Work out the finished part from the listing and answer in its coordinate system (mm). A direction names the side the tool comes from. Round coordinates to 2 decimals unless told otherwise and drop trailing zeros. Order: outer loops, then holes, each group sorted by start corner. A loop starts at its lowest first (then second) coordinate and runs counter-clockwise, first axis right, second up. Notation, with made-up numbers: (84, 80) - (119, 80) arc R6 ccw to (119, 87) - close; hole circle Ø11 at (13, -37). An arc over 180 degrees is marked (long way). Use one line per item in the form item = value. Start each with the question number.
Q1. The part is cut by section D-D on z = -6.75. Determine the outline of the cut face in (x, y).
Q2. The part is cut by section A-A on y = 12.9. Determine the outline of the cut face in (x, z).
Q3. Which of the six approach directions +Z, -Z, +X, -X, +Y, -Y give full straight-line access (tool end or side, diameter ignored) to faces 1 (the flat face through (0, -11.25, -5)), 2 (the flat face through (-12, -1, -5)), 3 (the flat face through (-10, -1, -6))?
Q4. The part is cut by section C-C on x = 68.1. Determine the outline of the cut face in (y, z), plus the area to 3 significant figures.
Q5. The part is cut by section B-B on x = -0.9. State how many separate pieces and enclosed holes the cut face has, plus the area to 3 significant figures.
Q6. Find the intervals of material crossed by line 1 (Y direction, x = -0.9, z = 0.3); line 2 (Y direction, x = -0.9, z = 0.45); line 3 (Z direction, x = -17, y = 17), in increasing order. Write a range as [from, to].
Q7. Given P1, Ø11.5, axis at x = -29.5, y = -8, coming from the -Z side; P2, Ø1, axis at y = -2, z = -4, coming from the -X side; P3, Ø1, axis at y = 8.5, z = -5.5, coming from the +X side, each flat-ended and moving along its own axis, determine where each tip first touches the part or whether it passes through.
Q8. For a pull along Y with two mould halves and no side action, classify faces 4 (the cylindrical face through (-1.28, -16.81, 0.51)), 5 (the flat face through (0, 8.25, -5)), 6 (the flat face through (12, 0.7, -8.9)) as +Y half, -Y half, draft (parallel to the pull), parting line (faces both ways), or undercut.
from build123d import *

# Parameters (mm, degrees)
SKETCH_W           = 151.8
SKETCH_H           = 41.8
PAD_DEPTH          = 2
CHAMFER_SIZE       = 1.9
SKETCH001_W        = 2
SKETCH001_H        = 2
PAD001_DEPTH       = 8.6
SKETCH002_W        = 15.5
SKETCH002_H        = 2
POCKET_DEPTH       = 2
SKETCH003_W        = 24
SKETCH003_H        = 19.5
PAD002_DEPTH       = 2
PAD003_START       = -0.75
SKETCH004_W        = 8
SKETCH004_H        = 0.6
PAD003_DEPTH       = 0.5
CHAMFER001_1_ANGLE = 53
CHAMFER001_1_SIZE  = 0.55
CHAMFER001_2_ANGLE = 53
CHAMFER001_2_SIZE  = 0.55
FILLET_R           = 1
FILLET001_R        = 1
SKETCH005_R        = 1.75
POCKET001_DEPTH    = 3
CHAMFER002_SIZE    = 1
SKETCH006_W        = 15.5
SKETCH006_H        = 8.6
POCKET002_DEPTH    = 5
SKETCH007_W        = 20
SKETCH007_H        = 15.5
POCKET003_DEPTH    = 5
SKETCH008_W        = 26
SKETCH008_H        = 21.5
POCKET004_DEPTH    = 10.6
SKETCH009_W        = 24
SKETCH009_H        = 19.5
SKETCH009_W_2      = 20
SKETCH009_H_2      = 15.5
PAD004_DEPTH       = 10.6
SKETCH010_W        = 15.5
SKETCH010_H        = 8.6
POCKET005_DEPTH    = 5
SKETCH011_W        = 15.5
SKETCH011_H        = 2
POCKET006_DEPTH    = 5
FILLET002_R        = 1.5


with BuildPart() as part:
    # Sketch → Pad (new body)
    with BuildSketch(Plane.XY):
        Rectangle(SKETCH_W, SKETCH_H)
    extrude(amount=PAD_DEPTH)

    # Chamfer
    chamfer_edges = [part.edges().sort_by_distance(p)[0] for p in [
        (0, -20.9, 0),
        (-75.9, 0, 0),
        (0, 20.9, 0),
        (75.9, 0, 0),
    ]]
    chamfer(chamfer_edges, length=CHAMFER_SIZE)

    # Sketch001 (on Face8 of Chamfer) → Pad001 (join)
    with BuildSketch(Plane(origin=(0, 0, 0), x_dir=(1, 0, 0), z_dir=(0, 0, -1))):
        Polygon((-11, 7.75), (-9, 7.75), (-9, 9.75), (-13, 9.75), (-13, -9.75), (-9, -9.75), (-9, -7.75), (-11, -7.75), align=None)
        with Locations((10, 8.75)):
            Rectangle(SKETCH001_W, SKETCH001_H)
        with Locations((10, -8.75)):
            Rectangle(SKETCH001_W, SKETCH001_H)
    extrude(amount=PAD001_DEPTH)

    # Sketch002 (on Face19 of Pad001) → Pocket (cut)
    with BuildSketch(Plane(origin=(-13, 0, 0), x_dir=(0, -1, 0), z_dir=(-1, 0, 0))):
        with Locations((0, -1)):
            Rectangle(SKETCH002_W, SKETCH002_H)
    extrude(amount=-POCKET_DEPTH, mode=Mode.SUBTRACT)

    # Sketch003 (on Face31 of Pocket) → Pad002 (join)
    with BuildSketch(Plane(origin=(0, 0, -8.6), x_dir=(1, 0, 0), z_dir=(0, 0, -1))):
        with Locations((-1, 0)):
            Rectangle(SKETCH003_W, SKETCH003_H)
        Polygon((-11, 7.75), (-1.5, 0), (-11, -7.75), align=None, mode=Mode.SUBTRACT)
        Polygon((9, 7.75), (1.5, 0), (9, -7.75), align=None, mode=Mode.SUBTRACT)
        Polygon((7, -7.75), (0, -1.5), (-9, -7.75), align=None, mode=Mode.SUBTRACT)
        Polygon((-9, 7.75), (0, 1.5), (7, 7.75), align=None, mode=Mode.SUBTRACT)
    extrude(amount=PAD002_DEPTH)

    # Sketch004 (on Face34 of Pad002) → Pad003 (join)
    with BuildSketch(Plane.YZ.offset(11).offset(PAD003_START)):
        with Locations((0, -8.3)):
            Rectangle(SKETCH004_W, SKETCH004_H)
    extrude(amount=-PAD003_DEPTH)

    # Chamfer001 1
    chamfer001_1_edges = [part.edges().sort_by_distance(p)[0] for p in [
        (10.25, 0, -8.6),
    ]]
    chamfer001_1_side = part.faces().sort_by_distance((10.25, 0, -8.3))[0]
    chamfer(chamfer001_1_edges, length=CHAMFER001_1_SIZE, angle=CHAMFER001_1_ANGLE, reference=chamfer001_1_side)

    # Chamfer001 2
    chamfer001_2_edges = [part.edges().sort_by_distance(p)[0] for p in [
        (9.75, 0, -8.6),
    ]]
    chamfer001_2_side = part.faces().sort_by_distance((9.75, 0, -8.3))[0]
    chamfer(chamfer001_2_edges, length=CHAMFER001_2_SIZE, angle=CHAMFER001_2_ANGLE, reference=chamfer001_2_side)

    # Fillet
    fillet_edges = [part.edges().sort_by_distance(p)[0] for p in [
        (10, -9.75, 0),
        (11, -8.75, 0),
        (9, -8.75, 0),
        (9, 8.75, 0),
        (10, 9.75, 0),
        (11, 8.75, 0),
        (-11, -9.75, 0),
        (-9, -8.75, 0),
        (-13, -8.75, 0),
        (-13, 8.75, 0),
        (-11, 9.75, 0),
        (-9, 8.75, 0),
        (11, -9.75, -5.3),
        (11, 9.75, -5.3),
        (-13, 9.75, -5.3),
        (-13, -9.75, -5.3),
    ]]
    fillet(fillet_edges, radius=FILLET_R)

    # Fillet001
    fillet001_edges = [part.edges().sort_by_distance(p)[0] for p in [
        (10.707107, -9.457107, -10.6),
    ]]
    fillet(fillet001_edges, radius=FILLET001_R)

    # Sketch005 (on Face73 of Fillet001) → Pocket001 (cut)
    with BuildSketch(Plane.XY.offset(2)):
        with Locations((-69.9, -1.1)):
            Circle(SKETCH005_R)
        with Locations((68.1, -0.1)):
            Circle(SKETCH005_R)
        with Locations((-0.9, -15.1)):
            Circle(SKETCH005_R)
        with Locations((-0.9, 12.9)):
            Circle(SKETCH005_R)
    extrude(amount=-POCKET001_DEPTH, mode=Mode.SUBTRACT)

    # Chamfer002
    chamfer002_edges = [part.edges().sort_by_distance(p)[0] for p in [
        (-2.65, 12.9, 2),
        (-71.65, -1.1, 2),
        (-2.65, -15.1, 2),
        (66.35, -0.1, 2),
    ]]
    chamfer(chamfer002_edges, length=CHAMFER002_SIZE)

    # Sketch006 (on Face46 of Chamfer002) → Pocket002 (cut)
    with BuildSketch(Plane.YZ.offset(11)):
        with Locations((0, -4.3)):
            Rectangle(SKETCH006_W, SKETCH006_H)
    extrude(amount=-POCKET002_DEPTH, mode=Mode.SUBTRACT)

    # Sketch007 (on Face59 of Pocket002) → Pocket003 (cut)
    with BuildSketch(Plane(origin=(0, 0, -10.6), x_dir=(1, 0, 0), z_dir=(0, 0, -1))):
        with Locations((-1, 0)):
            Rectangle(SKETCH007_W, SKETCH007_H)
    extrude(amount=-POCKET003_DEPTH, mode=Mode.SUBTRACT)

    # Sketch008 (on Face58 of Pocket003) → Pocket004 (cut)
    with BuildSketch(Plane(origin=(0, 0, -10.6), x_dir=(1, 0, 0), z_dir=(0, 0, -1))):
        with Locations((-1, 0)):
            Rectangle(SKETCH008_W, SKETCH008_H)
    extrude(amount=-POCKET004_DEPTH, mode=Mode.SUBTRACT)

    # Sketch009 (on Face18 of Pocket004) → Pad004 (join)
    with BuildSketch(Plane(origin=(0, 0, 0), x_dir=(1, 0, 0), z_dir=(0, 0, -1))):
        with Locations((0, 1.5)):
            Rectangle(SKETCH009_W, SKETCH009_H)
        with Locations((0, 1.5)):
            Rectangle(SKETCH009_W_2, SKETCH009_H_2, mode=Mode.SUBTRACT)
    extrude(amount=PAD004_DEPTH)

    # Sketch010 (on Face11 of Pad004) → Pocket005 (cut)
    with BuildSketch(Plane.YZ.offset(12)):
        with Locations((-1.5, -4.3)):
            Rectangle(SKETCH010_W, SKETCH010_H)
    extrude(amount=-POCKET005_DEPTH, mode=Mode.SUBTRACT)

    # Sketch011 (on Face31 of Pocket005) → Pocket006 (cut)
    with BuildSketch(Plane.YZ.offset(-10)):
        with Locations((-1.5, -1)):
            Rectangle(SKETCH011_W, SKETCH011_H)
    extrude(amount=-POCKET006_DEPTH, mode=Mode.SUBTRACT)

    # Fillet002
    fillet002_edges = [part.edges().sort_by_distance(p)[0] for p in [
        (12, -10.25, 0),
        (0, -11.25, 0),
        (-12, -10.25, 0),
        (0, 8.25, 0),
        (12, 7.25, 0),
        (12, -1.5, -10.6),
        (0, 8.25, -10.6),
        (-12, -1.5, -10.6),
        (0, -11.25, -10.6),
        (-12, 7.25, 0),
    ]]
    fillet(fillet002_edges, radius=FILLET002_R)


solid = part.part
Found:
q1.outline = (-12, -11.25) - (12, -11.25) - (12, -9.25) - (-10, -9.25) - (-10, 6.25) - (12, 6.25) - (12, 8.25) - (-12, 8.25) - close
q2.outline = (-75.9, 1.9) - (-74, 0) - (-2.65, 0) - (-2.65, 1) - (-3.65, 2) - (-75.9, 2) - close; (0.85, 0) - (74, 0) - (75.9, 1.9) - (75.9, 2) - (1.85, 2) - (0.85, 1) - close
q3.face_1 = -Z, +X, -X, -Y
q3.face_2 = -Z, -X, +Y, -Y
q3.face_3 = -Z
q4.outline = (-20.9, 1.9) - (-19, 0) - (-1.85, 0) - (-1.85, 1) - (-2.85, 2) - (-20.9, 2) - close; (1.65, 0) - (19, 0) - (20.9, 1.9) - (20.9, 2) - (2.65, 2) - (1.65, 1) - close
q4.area = 72.0 mm²
q5.separate_pieces = 3
q5.enclosed_holes = 0
q5.area = 106 mm²
q6.line_1 = [-19.3, -16.85], [-13.35, 11.15], [14.65, 19.3]
q6.line_2 = [-19.45, -16.85], [-13.35, 11.15], [14.65, 19.45]
q6.line_3 = [0, 2]
q7.P1 = 0
q7.P2 = -12
q7.P3 = 12
q8.face_4 = undercut
q8.face_5 = +Y half
q8.face_6 = draft
